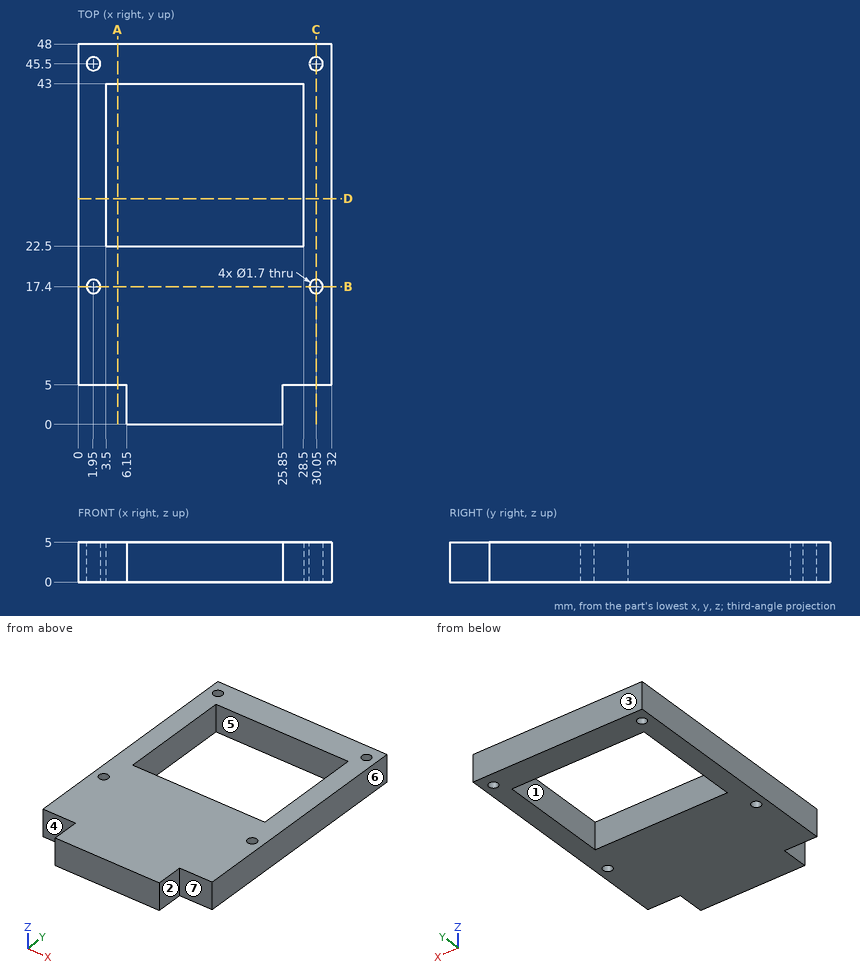
Job drawing, mm, ordinate dimensions from the low corner. One solid piece. A direction names the side the tool comes from. Round coordinates to 2 decimals unless told otherwise and drop trailing zeros. Write each loop counter-clockwise with the first axis right and the second up, starting at its lowest first coordinate (ties: lowest second). Pieces come first, ordered by that corner, then holes.
1) Band-saw the part on B-B, the plane y = 17.4. List the corners of the cut face in (x, z), and give its area (3 significant figures).
2) Band-saw the part on A-A, the plane x = 5. List the corners of the cut face in (y, z).
3) Mould opens along X. For the marked faces 1, 2 and 3 say: +X half, -X half, draft (parallel to the pull), parting line (faces both ways), or undercut.
4) Band-saw the part on C-C, the plane x = 30.05. List the corners of the cut face in (y, z).
5) Drill centre lines: probe 1 along Y at (x, z) = (1.95, 1.5); probe 2 along X at (y, z) = (45.5, 1.8); probe 3 along X at (y, z) = (41.5, 3.4). Where is each one in solid material? Low to high.
6) 3-axis set-ups, long thin cutter, end or side, ignore diameter. For the marked faces 4, 5, 6 and 7: which of +Z, -Z, +X, -X, +Y, -Y reach the whole face in a straight line?
7) Pin check, flat tips, straight feed: pin 1 (1.5 mm diameter, centred on y = 3, z = 3.5, fed in from +X); pin 2 (1.5 mm diameter, centred on x = 2.5, z = 1.5, fed in from -Y). Stop position of each tip, or through.
8) Band-saw the part on D-D, the plane y = 28.5. List the corners of the cut face in (x, z), and give its area (3 significant figures).
Ans:
1. outline: (0, 0) - (1.1, 0) - (1.1, 5) - (0, 5) - close; (2.8, 0) - (29.2, 0) - (29.2, 5) - (2.8, 5) - close; (30.9, 0) - (32, 0) - (32, 5) - (30.9, 5) - close
1. area: 143 mm2
2. outline: (5, 0) - (22.5, 0) - (22.5, 5) - (5, 5) - close; (43, 0) - (48, 0) - (48, 5) - (43, 5) - close
3. face 1: undercut
3. face 2: +X half
3. face 3: draft
4. outline: (5, 0) - (16.55, 0) - (16.55, 5) - (5, 5) - close; (18.25, 0) - (44.65, 0) - (44.65, 5) - (18.25, 5) - close; (46.35, 0) - (48, 0) - (48, 5) - (46.35, 5) - close
5. probe 1: y = 5 to 16.55, 18.25 to 44.65, 46.35 to 48
5. probe 2: x = 0 to 1.1, 2.8 to 29.2, 30.9 to 32
5. probe 3: x = 0 to 3.5, 28.5 to 32
6. face 4: +Z, -Z, -X, -Y
6. face 5: +Z, -Z
6. face 6: +Z, -Z, +X, +Y, -Y
6. face 7: +Z, -Z, +X, -Y
7. pin 1: stops at x = 25.85
7. pin 2: stops at y = 5
8. outline: (0, 0) - (3.5, 0) - (3.5, 5) - (0, 5) - close; (28.5, 0) - (32, 0) - (32, 5) - (28.5, 5) - close
8. area: 35.0 mm2
